Print and shaded views of the part. All mm, measured from the part's lowest x, y and z. A direction names the side the tool comes from. Coordinates: 2 decimals unless noted, no trailing zeros. Loops run counter-clockwise (first coordinate to the right, second up) from the corner with the lowest first, then second, coordinate; pieces in that order, holes last. Notation, with made-up numbers: M 61,15.5 L 75,15.5 A8 cw 75,21.5 Z; hole C 64.5,68.5 d3. An arc over 180 degrees is marked long. Use a Markdown table: item, result. Add a question column.
1) Wall check: probe 1 along Y at (x, z) = (10, 13.5); probe 2 along X at (y, z) = (3.5, 28.5); probe 3 along X at (y, z) = (8.25, 16.5). Give the ranges that are in metal, low to high. Write a range as from..to.
2) Band-saw the part on B-B (x = 21). List the corners of the cut face in (y, z).
3) Band-saw the part on A-A (z = 17.5). List the corners of the cut face in (x, y), plus the area to 3 significant figures.
4) Tool access for the marked faces 1 and 2: list every direction of +Z, -Z, +X, -X, +Y, -Y with a clear straight run to the whole face (end or side of a thin tool).
5) Pin check, flat tips, straight feed: pin 1 Ø3 at (x, y) = (14.5, 11.5) entering from +Z; pin 2 Ø1.5 at (y, z) = (5.5, 10.5) entering from +X; pin 3 Ø3 at (y, z) = (8.5, 13.5) entering from -X. Stop position of each tip, or through.
6) Pull direction Z, two halves, no side cores. Call the marked faces 3, 4 and 5: released by +Z, released by -Z, zero draft, split by the parting line, or undercut.
7) Band-saw the part on D-D (y = 19.5). List the corners of the cut face in (x, z).
8) Band-saw the part on C-C (x = 17.5). List the corners of the cut face in (y, z), plus the area to 3 significant figures.
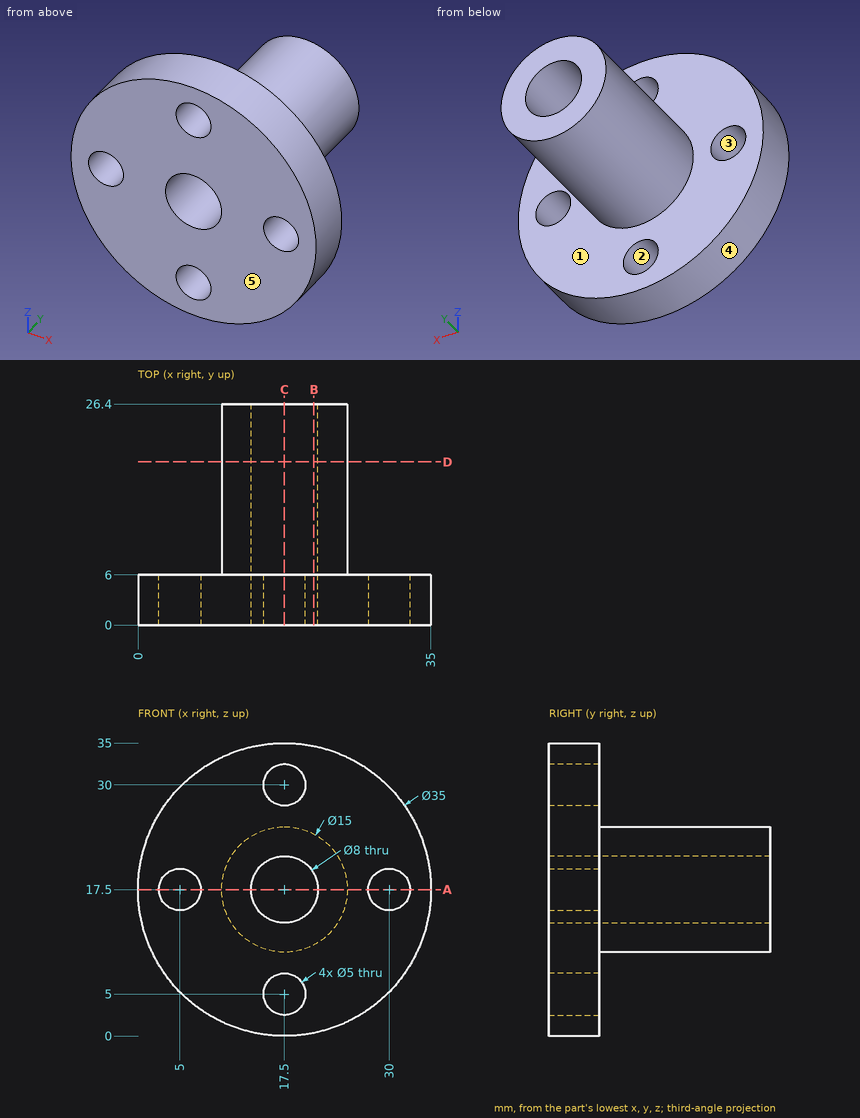
Entries:
| question | item | result |
|---|---|---|
| 1 | probe 1 | 0..6 |
| 1 | probe 2 | 3.89..15.5, 19.5..31.11 |
| 1 | probe 3 | 10.07..13.63, 21.37..24.93 |
| 2 | outline | M 0,0.35 L 6,0.35 L 6,10.87 L 26.4,10.87 L 26.4,15.56 L 0,15.56 Z; M 0,19.44 L 26.4,19.44 L 26.4,24.13 L 6,24.13 L 6,34.65 L 0,34.65 Z |
| 3 | outline | M 0,0 L 2.5,0 L 2.5,6 L 0,6 Z; M 7.5,0 L 13.5,0 L 13.5,26.4 L 10,26.4 L 10,6 L 7.5,6 Z; M 21.5,0 L 27.5,0 L 27.5,6 L 25,6 L 25,26.4 L 21.5,26.4 Z; M 32.5,0 L 35,0 L 35,6 L 32.5,6 Z |
| 3 | area | 245 mm2 |
| 4 | face 1 | +Y |
| 4 | face 2 | +Y, -Y |
| 5 | pin 1 | z = 24.85 |
| 5 | pin 2 | x = 33.85 |
| 5 | pin 3 | x = 10.43 |
| 6 | face 3 | undercut |
| 6 | face 4 | split by the parting line |
| 6 | face 5 | zero draft |
| 7 | outline | C 17.5,17.5 d15; hole C 17.5,17.5 d8 |
| 8 | outline | M 0,0 L 6,0 L 6,2.5 L 0,2.5 Z; M 0,7.5 L 6,7.5 L 6,10 L 26.4,10 L 26.4,13.5 L 0,13.5 Z; M 0,21.5 L 26.4,21.5 L 26.4,25 L 6,25 L 6,27.5 L 0,27.5 Z; M 0,32.5 L 6,32.5 L 6,35 L 0,35 Z |
| 8 | area | 245 mm2 |
